Here's how the part is built. I have some questions about the finished solid (model axes, mm). A direction names the side the tool comes from. Round coordinates to 2 decimals unless told otherwise and drop trailing zeros. Loops run counter-clockwise (first coordinate to the right, second up) from the corner with the lowest first, then second, coordinate; pieces in that order, holes last. Notation, with made-up numbers: (53.25, 82) -> (94.25, 82) arc R9 ccw to (94.25, 94) -> close; hole circle Ø11 at (-23.75, 41.25). An arc over 180 degrees is marked (long way). Use one line per item in the form item = value. Start each with the question number.
Item 1: I'm going to push flat-ended pins straight in: pin 1 Ø3 at (y, z) = (11.5, 6) entering from +X; pin 2 Ø1 at (y, z) = (6.5, 45.5) entering from -X; pin 3 Ø6 at (y, z) = (9, 11.5) entering from -X. Where does each tip first touch, or does it pass through?
Item 2: If I drill on L1, parallel to Y at x = 0, z = 2; L2, parallel to Z at x = -8.5, y = -9; L3, parallel to Y at x = 0, z = -0.25, over which ranges is the centre line in solid material (lowest first)? Write a range as [from, to].
Item 3: If we section it at C-C (x = 8.5): Write out the boundary of the cut face in (y, z), then the cut area to 3 significant figures.
Item 4: If we section it at A-A (y = 0): Write out the boundary of the cut face in (x, z) (3 decimals).
Item 5: If we section it at B-B (z = 44): Write out the boundary of the cut face in (x, y), then the cut area to 3 significant figures.
Item 6: Thinking about a two-plate mould opening in Y: for faces 1 (the face through (3, -10, -4)), 2 (the face through (-1.301, -4.143, -1.972)), 3 (the face through (0, 0, 47)), which applies, released by +Y, released by -Y, zero draft, split by the parting line, or undercut?
Item 7: For faces 4 (the face through (0.54, -12.44, 0.56)), 5 (the face through (6.759, 6, 44)), 6 (the face through (-6.759, -6, 44)), 7 (the face through (0.1, 10.13, 44.46)), which set-ups out of +Z, -Z, +X, -X, +Y, -Y let a thin tool reach every point of the face, with its end or its side?
Item 8: If we section it at D-D (x = 0): Write out the boundary of the cut face in (y, z) (3 decimals), then the cut area to 3 significant figures.
```python
from build123d import *

# Parameters (mm, degrees)
SKETCH1_R           = 17.5
BOSS_EXTRUDE1_DEPTH = 20
SKETCH2_R           = 13.371126373
BOSS_EXTRUDE2_DEPTH = 22
BOSS_EXTRUDE3_DEPTH = 5
SKETCH4_R           = 12.665000137
BOSS_EXTRUDE4_DEPTH = 2
SKETCH5_R           = 2.5
BOSS_EXTRUDE5_DEPTH = 20
SKETCH6_R           = 6
SKETCH6_R_2         = 2.5
BOSS_EXTRUDE6_DEPTH = 4
CUT_EXTRUDE1_START  = -25
SKETCH8_R           = 2.5
CUT_EXTRUDE1_DEPTH  = 25


with BuildPart() as part:
    # Sketch1 → Boss-Extrude1 (new body)
    with BuildSketch(Plane.XY):
        Circle(SKETCH1_R)
    extrude(amount=BOSS_EXTRUDE1_DEPTH)

    # Sketch2 → Boss-Extrude2 (add)
    with BuildSketch(Plane.XY.offset(20)):
        Circle(SKETCH2_R)
    extrude(amount=BOSS_EXTRUDE2_DEPTH)

    # Sketch3 → Boss-Extrude3 (add)
    with BuildSketch(Plane.XY.offset(42)):
        with BuildLine():
            Line((-6.759376189, 7.547571999), (-6.759376189, 5.4522877))
            ThreePointArc((-6.759376189, 5.4522877), (0, 8.684273581), (6.759376189, 5.4522877))
            Line((6.759376189, 5.4522877), (6.759376189, 7.547571999))
            ThreePointArc((6.759376189, 7.547571999), (0, 10.131880849), (-6.759376189, 7.547571999))
        make_face()
        with BuildLine():
            Line((-6.759376189, -5.4522877), (-6.759376189, -7.547571999))
            ThreePointArc((-6.759376189, -7.547571999), (0, -10.131880849), (6.759376189, -7.547571999))
            Line((6.759376189, -7.547571999), (6.759376189, -5.4522877))
            ThreePointArc((6.759376189, -5.4522877), (0, -8.684273581), (-6.759376189, -5.4522877))
        make_face()
    extrude(amount=BOSS_EXTRUDE3_DEPTH)

    # Sketch4 → Boss-Extrude4 (add)
    with BuildSketch(Plane.XY.offset(47)):
        Circle(SKETCH4_R)
    extrude(amount=BOSS_EXTRUDE4_DEPTH)

    # Sketch5 → Boss-Extrude5 (add)
    with BuildSketch(Plane(origin=(0, 0, 0), x_dir=(-1, 0, 0), z_dir=(0, 0, -1))):
        with Locations(Location((0, -10, 0), (0, 0, 180))):
            Circle(SKETCH5_R)
    extrude(amount=BOSS_EXTRUDE5_DEPTH)

    # Sketch6 → Boss-Extrude6 (add)
    with BuildSketch(Plane(origin=(0, 0, 0), x_dir=(-1, 0, 0), z_dir=(0, 0, -1))):
        with Locations(Location((0, -10, 0), (0, 0, 180))):
            Circle(SKETCH6_R)
        with Locations((0, -10)):
            Circle(SKETCH6_R_2, mode=Mode.SUBTRACT)
    extrude(amount=BOSS_EXTRUDE6_DEPTH)

    # Sketch8 → Cut-Extrude1 (cut)
    with BuildSketch(Plane(origin=(0, 0, -20), x_dir=(-1, 0, 0), z_dir=(0, 0, -1)).offset(CUT_EXTRUDE1_START)):
        with Locations((0, -10)):
            Circle(SKETCH8_R)
    extrude(amount=CUT_EXTRUDE1_DEPTH, mode=Mode.SUBTRACT)


solid = part.part
```
Values found:
q1.pin_1 = 14.36
q1.pin_2 = -6.76
q1.pin_3 = -16.44
q2.L1 = [-17.5, -12.5], [-7.5, 17.5]
q2.L2 = [0, 42], [47, 49]
q2.L3 = [-16, -12.5], [-7.5, -4]
q3.outline = (-15.3, 0) -> (15.3, 0) -> (15.3, 20) -> (10.32, 20) -> (10.32, 42) -> (-10.32, 42) -> (-10.32, 20) -> (-15.3, 20) -> close; (-9.39, 47) -> (9.39, 47) -> (9.39, 49) -> (-9.39, 49) -> close
q3.area = 1,100 mm2
q4.outline = (-17.5, 0) -> (17.5, 0) -> (17.5, 20) -> (13.371, 20) -> (13.371, 42) -> (-13.371, 42) -> (-13.371, 20) -> (-17.5, 20) -> close; (-12.665, 47) -> (12.665, 47) -> (12.665, 49) -> (-12.665, 49) -> close
q5.outline = (-6.76, -7.55) arc R10.13 ccw to (6.76, -7.55) -> (6.76, -5.45) arc R8.68 cw to (-6.76, -5.45) -> close; (-6.76, 5.45) arc R8.68 cw to (6.76, 5.45) -> (6.76, 7.55) arc R10.13 ccw to (-6.76, 7.55) -> close
q5.area = 43.7 mm2
q6.face_1 = zero draft
q6.face_2 = split by the parting line
q6.face_3 = undercut
q7.face_4 = -Z
q7.face_5 = +X, +Y, -Y
q7.face_6 = -X, +Y, -Y
q7.face_7 = +Y
q8.outline = (-17.5, 0) -> (-16, 0) -> (-16, -4) -> (-12.5, -4) -> (-12.5, 5) -> (-7.5, 5) -> (-7.5, -4) -> (-4, -4) -> (-4, 0) -> (17.5, 0) -> (17.5, 20) -> (13.371, 20) -> (13.371, 42) -> (10.132, 42) -> (10.132, 47) -> (12.665, 47) -> (12.665, 49) -> (-12.665, 49) -> (-12.665, 47) -> (-10.132, 47) -> (-10.132, 42) -> (-13.371, 42) -> (-13.371, 20) -> (-17.5, 20) -> close; hole (-8.684, 42) -> (8.684, 42) -> (8.684, 47) -> (-8.684, 47) -> close
q8.area = 1,360 mm2
